The listing builds one solid part. Answer for the finished solid, in the listing's coordinates (mm). Give positions to 0.01 mm unless a question says otherwise; leave off trailing zeros. Order: outer loops, then holes, each group sorted by start corner. A loop starts at its lowest first (then second) coordinate and runs counter-clockwise, first axis right, second up. Notation, with made-up numbers: (-5.5, -15) -> (33.5, -15) arc R15 cw to (33.5, -3) -> close; hole circle Ø9 at (-9.75, 58). An arc over 180 degrees is marked (long way). Write item = value, one per line. Start each with the question number.
```python
from build123d import *

# Parameters (mm, degrees)
F0_W         = 6.35
F0_H         = 6.35
F0_H_2       = 1466.85
F1_DEPTH     = 3.175
F2_R         = 3.175
F3_DEPTH     = 12.7
F4_T3_DEPTH  = 1489.075
F4_S4_R      = 3.175
F4_T5_DEPTH  = 746
F4_T8_DEPTH  = 1489.075
F4_S9_R      = 3.175
F4_T10_DEPTH = 746
F4_T13_DEPTH = 1489.075
F4_S14_R     = 3.175
F4_T15_DEPTH = 746
F4_T18_DEPTH = 1489.075
F4_S19_R     = 3.175
F4_T20_DEPTH = 746


# Not quite as in the source:
# - a fillet or chamfer that OpenCascade refuses, or shapes differently, is made with other operations: its cross-section is extruded or revolved along the edge and cut away or added


with BuildPart() as f1:
    # F0 (on Front) → F1 (new body, symmetric)
    with BuildSketch(Plane.XZ):
        with Locations((0, 733.425)):
            Rectangle(F0_W, F0_H)
        with Locations((0, -3.175)):
            Rectangle(F0_W, F0_H_2)
    extrude(amount=F1_DEPTH, both=True)

    # F2 (on Front) → F3 (join, symmetric)
    with BuildSketch(Plane.XZ):
        with Locations((0, 736.6)):
            Circle(F2_R)
    extrude(amount=F3_DEPTH, both=True)

    # F4: fillet of radius 3.175 on 4 edges, made by hand


with BuildPart() as f4_tool1:
    # F4_s2 → F4_t3 (new body)
    with BuildSketch(Plane.XY.offset(-744.5375)):
        with BuildLine():
            ThreePointArc((0, -3.175), (2.2450640303, -2.2450640303), (3.175, 0))
            Line((3.175, 0), (3.175, -3.175))
            Line((3.175, -3.175), (0, -3.175))
        make_face()
    extrude(amount=F4_T3_DEPTH)

    # F4_s4 → F4_t5 (cut, symmetric)
    with BuildSketch(Plane.XZ.offset(1.6)):
        with Locations((0, 736.6)):
            Circle(F4_S4_R)
    extrude(amount=F4_T5_DEPTH, both=True, mode=Mode.SUBTRACT)


with BuildPart() as f4_tool6:
    # F4_s7 → F4_t8 (new body)
    with BuildSketch(Plane.XY.offset(-744.5375)):
        with BuildLine():
            ThreePointArc((0, 3.175), (2.2450640303, 2.2450640303), (3.175, 0))
            Line((3.175, 0), (3.175, 3.175))
            Line((3.175, 3.175), (0, 3.175))
        make_face()
    extrude(amount=F4_T8_DEPTH)

    # F4_s9 → F4_t10 (cut, symmetric)
    with BuildSketch(Plane.XZ.offset(-1.6)):
        with Locations((0, 736.6)):
            Circle(F4_S9_R)
    extrude(amount=F4_T10_DEPTH, both=True, mode=Mode.SUBTRACT)


with BuildPart() as f4_tool11:
    # F4_s12 → F4_t13 (new body)
    with BuildSketch(Plane.XY.offset(744.5375)):
        with BuildLine():
            ThreePointArc((-3.175, 0), (-2.2450640303, 2.2450640303), (0, 3.175))
            Line((0, 3.175), (-3.175, 3.175))
            Line((-3.175, 3.175), (-3.175, 0))
        make_face()
    extrude(amount=-F4_T13_DEPTH)

    # F4_s14 → F4_t15 (cut, symmetric)
    with BuildSketch(Plane.XZ.offset(-1.6)):
        with Locations((0, 736.6)):
            Circle(F4_S14_R)
    extrude(amount=F4_T15_DEPTH, both=True, mode=Mode.SUBTRACT)


with BuildPart() as f4_tool16:
    # F4_s17 → F4_t18 (new body)
    with BuildSketch(Plane.XY.offset(744.5375)):
        with BuildLine():
            ThreePointArc((-3.175, 0), (-2.2450640303, -2.2450640303), (0, -3.175))
            Line((0, -3.175), (-3.175, -3.175))
            Line((-3.175, -3.175), (-3.175, 0))
        make_face()
    extrude(amount=-F4_T18_DEPTH)

    # F4_s19 → F4_t20 (cut, symmetric)
    with BuildSketch(Plane.XZ.offset(1.6)):
        with Locations((0, 736.6)):
            Circle(F4_S19_R)
    extrude(amount=F4_T20_DEPTH, both=True, mode=Mode.SUBTRACT)


with BuildPart() as f1_1:
    add(f1.part)

    # F4_t21: cut F4_tool1, F4_tool6, F4_tool11, F4_tool16
    add([f4_tool1.part, f4_tool6.part, f4_tool11.part, f4_tool16.part], mode=Mode.SUBTRACT)


solid = f1_1.part
```
Item 1: Consider L1, parallel to Y at x = 0, z = 234.5 (3 decimals); L2, parallel to X at y = 0.25, z = -191.5; L3, parallel to X at y = -0.75, z = -54.5. Determine where each line is inside the solid, lowest interval first. Write a range as from..to.
Item 2: A cutting plane is placed at C-C, the plane y = -7.5. Write down the section's boundary in (x, z) (3 decimals).
Item 3: A cutting plane is placed at B-B, the plane x = -1.5. Write down the section's boundary in (y, z), plus the area to 3 significant figures.
Item 4: A cutting plane is placed at A-A, the plane z = -426. Write down the section's boundary in (x, y) (3 decimals), plus the area to 3 significant figures.
Item 5: Flat-ended cylindrical pins translate along their axes: pin 1 (3 mm diameter, centred on x = 1, y = 9, fed in from -Z) (3 decimals); pin 2 (6 mm diameter, centred on y = 3.5, z = -23.5, fed in from +X); pin 3 (2 mm diameter, centred on x = -0.5, y = -5.5, fed in from +Z) (3 decimals); pin 4 (1 mm diameter, centred on x = 1.5, y = 9.5, fed in from -Z). Find the tip coordinate at first contact, or state that the pin passes through.
Check values:
q1.L1 = -3.175..3.175
q1.L2 = -3.17..3.17
q1.L3 = -3.09..3.09
q2.outline = circle Ø6.35 at (0, 736.6)
q3.outline = (-12.7, 733.8) -> (-2.8, 733.8) -> (-2.8, -736.6) -> (2.8, -736.6) -> (2.8, 733.8) -> (12.7, 733.8) -> (12.7, 739.4) -> (-12.7, 739.4) -> close
q3.area = 8,370 mm^2
q4.outline = circle Ø6.35 at (0, 0)
q4.area = 31.7 mm^2
q5.pin_1 = 733.425
q5.pin_2 = 3.14
q5.pin_3 = 739.775
q5.pin_4 = 733.59
